Source: CAD feature listing. Evaluate the final solid. Frame: model axes, mm. A direction names the side the tool comes from. Coordinates: 2 decimals unless noted, no trailing zeros. Order: outer loops, then holes, each group sorted by start corner. A loop starts at its lowest first (then second) coordinate and runs counter-clockwise, first axis right, second up.
Autodesk Inventor part; units mm, degrees
ref_plane "YZ Plane" through (0, 0, 0) normal (1, 0, 0) x (0, 1, 0)
ref_plane "XZ Plane" through (0, 0, 0) normal (0, 1, 0) x (-1, 0, 0)
ref_plane "XY Plane" through (0, 0, 0) normal (0, 0, 1) x (1, 0, 0)
sketch "Sketch1" plane through (0, 0, 0) normal (0, 0, 1) x (1, 0, 0)
  line L0 (0, 0) -> (465, 0)
  line L1 (465, 0) -> (465, 377)
  line L2 (465, 377) -> (0, 377)
  line L3 (0, 377) -> (0, 0)
  line L4 (0, 188.5) -> (465, 188.5) construction
  line L5 (150, 478.4047) -> (150, -123.5436) construction
  circle A0 centre (150, 188.5) radius 42.3
  dimension "d0" = 465
  dimension "d1" = 377
  dimension "d7" = 315
  dimension "d8" = 84.6
extrude "Extrusion1" add sketch "Sketch1" along normal blind 3
sketch "Sketch2" plane through (0, 0, 0) normal (0, 0, -1) x (-1, 0, 0)
  circle A0 centre (-150, 188.5) radius 42.3
  line L0 (-465, 377) -> (0, 377)
  line L1 (0, 377) -> (0, 0)
  line L2 (0, 0) -> (-465, 0)
  line L3 (-465, 0) -> (-465, 377)
extrude "Extrusion2" add sketch "Sketch2" along normal blind 106
sketch "Sketch3" plane through (0, 0, -106) normal (0, 0, -1) x (-1, 0, 0)
  circle A0 centre (-150, 188.5) radius 42.3
  circle A1 centre (-150, 188.5) radius 50.9763
extrude "Extrusion3" add sketch "Sketch3" against normal blind 10.9 contours A0
fillet "Fillet1" radius 120 4 edges at (465, 0, -51.5) (465, 377, -51.5) (0, 0, -51.5) (0, 377, -51.5)
sketch "Sketch4" plane through (0, 0, 3) normal (0, 0, 1) x (1, 0, 0)
  arc A0 (120, 377) -> (0, 257) centre (120, 257) ccw
  line L0 (0, 257) -> (0, 120)
  arc A1 (0, 120) -> (120, 0) centre (120, 120) ccw
  line L1 (120, 0) -> (345, 0)
  arc A2 (345, 0) -> (465, 120) centre (345, 120) ccw
  line L2 (465, 120) -> (465, 257)
  arc A3 (465, 257) -> (345, 377) centre (345, 257) ccw
  line L3 (345, 377) -> (120, 377)
  circle A4 centre (150, 188.5) radius 42.3
  point P0 (0, 0)
shell "Shell1" thickness 3 removed faces 1 at (195, 125.6667, -106)
properties part number "Pseudo-Guitar"
1. Draft query along Y for faces 1 (the face through (231, 3, -54)), 2 (the face through (0, 189, -52)), 3 (the face through (231, 0, -52)). Return one class per face: released by +Y, released by -Y, zero draft, split by the parting line, or undercut.
Findings:
face 1: undercut
face 2: zero draft
face 3: released by -Y
2. Section query B-B on x = 204.5. Return loops of the section in (y, z), plus the area to 3 significant figures.
Findings:
outline: (0, -106) - (3, -106) - (3, 0) - (374, 0) - (374, -106) - (377, -106) - (377, 3) - (0, 3) - close
area: 1,770 mm2
3. Pin query (flat end, axial travel): P1, Ø3, axis at y = 110.5, z = -85.5, coming from the +X side; P2, Ø10, axis at x = 378.5, z = -79.5, coming from the -Y side; P3, Ø1.5, axis at y = 296.5, z = -86, coming from the +X side. Return the tip coordinate at first contact, or that it passes through.
Findings:
P1: stops at x = 464.73
P2: stops at y = 3.43
P3: stops at x = 458.57
4. Access query for faces 4 (the face through (151, 189, -98.1)), 5 (the face through (234, 377, -52)), 6 (the face through (151, 189, -95.1)). Directions: +Z, -Z, +X, -X, +Y, -Y. A direction counts if a zero-diameter tool reaches every point of the face in a straight line with its end or side. Return the directions, or none.
Findings:
face 4: -Z
face 5: +Z, -Z, +X, -X, +Y
face 6: +Z
5. Section query A-A on z = -78. Return loops of the section in (x, y), plus the area to 3 significant figures.
Findings:
outline: (0, 120) arc R120 ccw to (120, 0) - (345, 0) arc R120 ccw to (465, 120) - (465, 257) arc R120 ccw to (345, 377) - (120, 377) arc R120 ccw to (0, 257) - close; circle Ø90.6 at (150, 188.5); hole (3, 120) arc R117 ccw to (120, 3) - (345, 3) arc R117 ccw to (462, 120) - (462, 257) arc R117 ccw to (345, 374) - (120, 374) arc R117 ccw to (3, 257) - close; hole circle Ø84.6 at (150, 188.5)
area: 5,230 mm2
6. Section query C-C on y = 245. Return loops of the section in (x, z).
Findings:
outline: (0, -106) - (3, -106) - (3, 0) - (462, 0) - (462, -106) - (465, -106) - (465, 3) - (0, 3) - close
7. Section query D-D on x = 150. Return loops of the section in (y, z).
Findings:
outline: (0, -106) - (3, -106) - (3, 0) - (143.2, 0) - (143.2, -98.1) - (233.8, -98.1) - (233.8, 0) - (374, 0) - (374, -106) - (377, -106) - (377, 3) - (230.8, 3) - (230.8, -95.1) - (146.2, -95.1) - (146.2, 3) - (0, 3) - close
8. Ray query, line 1 (X direction, y = 188, z = -42); line 2 (Y direction, x = 254.5, z = -28); line 3 (X direction, y = 188.5, z = 2.1). Return the intervals inside material, ascending.
Findings:
line 1: x = 0 to 3, 104.7 to 107.7, 192.3 to 195.3, 462 to 465
line 2: y = 0 to 3, 374 to 377
line 3: x = 0 to 107.7, 192.3 to 465
